The model under review builds one solid part; all positions refer to its coordinate system, in mm. Round coordinates to 2 decimals unless told otherwise and drop trailing zeros. Write each loop counter-clockwise with the first axis right and the second up, starting at its lowest first coordinate (ties: lowest second). Pieces come first, ordered by that corner, then holes. Notation, with made-up numbers: (-26.5, 52) -> (-15.5, 52) arc R11 ccw to (-15.5, 68) -> close; hole circle Ø4 at (-14, 46). An arc over 180 degrees is marked (long way). Return JSON: item names as keys, results as strings. Group by question number.
1. For line 1 along Y through (x, z) = (1, 0); line 2 along Z through (x, y) = (3.55, -1); line 3 along Y through (x, z) = (0.7, 3), list the stretches that pass through material, from the lowest coordinate up. Write a range as from..to.
2. Take a section at D-D, the plane z = -22. Write out the cut boundary in (x, y), then the cut area to 3 significant figures.
3. Take a section at B-B, the plane x = 2.1. Write out the cut boundary in (y, z), then the cut area to 3 significant figures.
4. Take a section at C-C, the plane y = 50. Write out the cut boundary in (x, z), then the cut area to 3 significant figures.
5. Take a section at A-A, the plane z = 0. Write out the cut boundary in (x, y), then the cut area to 3 significant figures.
6. Clearance check with a flat-ended pin moving along its axis: P1, Ø5, axis at y = 14.5, z = 44.5, coming from the -X side. State where the tip first meets the part, or that it passes through.
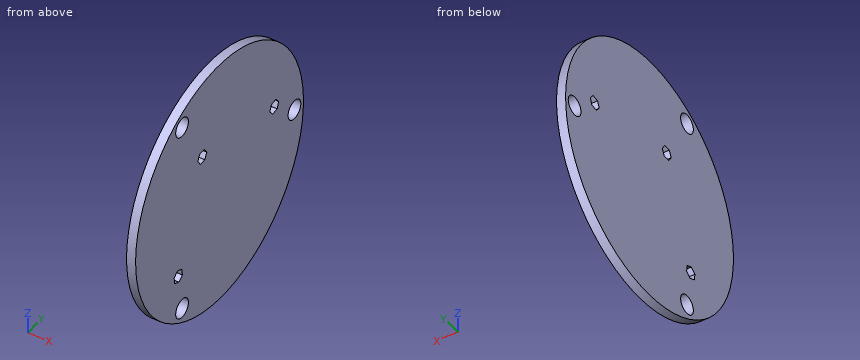
from build123d import *

# Parameters (mm, degrees)
SKETCH1_R           = 56
BOSS_EXTRUDE1_DEPTH = 4
SKETCH2_R           = 4.25
CUT_EXTRUDE1_DEPTH  = 80.296910406
CUT_EXTRUDE3_DEPTH  = 80.296910406


with BuildPart() as part:
    # Sketch1 → Boss-Extrude1 (new body)
    with BuildSketch(Plane(origin=(0, 0, 0), x_dir=(0, 0, -1), z_dir=(1, 0, 0))):
        Circle(SKETCH1_R)
    extrude(amount=BOSS_EXTRUDE1_DEPTH)

    # Sketch2 → Cut-Extrude1 (cut, through all)
    with BuildSketch(Plane.ZY):
        with Locations((0, 50)):
            Circle(SKETCH2_R)
        with Locations((43.301270189, -25)):
            Circle(SKETCH2_R)
        with Locations((-43.301270189, -25)):
            Circle(SKETCH2_R)
    extrude(amount=-CUT_EXTRUDE1_DEPTH, mode=Mode.SUBTRACT)

    # Sketch4 → Cut-Extrude3 (cut, through all)
    with BuildSketch(Plane(origin=(4, 0, 0), x_dir=(0, 0, -1), z_dir=(1, 0, 0))):
        Polygon((27.459399078, -24.776044357), (24.480611991, -25.150424944), (23.315441547, -27.917320527), (25.12905819, -30.309835523), (28.107845277, -29.935454936), (29.273015721, -27.168559353), align=None)
        Polygon((-13.023850584, 34.635102926), (-10.212575655, 33.581505942), (-7.894496437, 35.489342956), (-8.387692148, 38.450776954), (-11.198967077, 39.504373938), (-13.517046295, 37.596536924), align=None)
        Polygon((-17.236572945, -12.849128791), (-17.40919881, -9.85187444), (-20.091210152, -8.502745649), (-22.600595629, -10.150871209), (-22.427969764, -13.14812556), (-19.745958422, -14.497254351), align=None)
    extrude(amount=-CUT_EXTRUDE3_DEPTH, mode=Mode.SUBTRACT)


solid = part.part
Output:
{
 "1": {"line 1": "y = -56..45.75, 54.25..56", "line 2": "z = -55.99..55.99", "line 3": "y = -55.92..46.99, 53.01..55.92"},
 "2": {"outline": "(0, -51.5) -> (4, -51.5) -> (4, 51.5) -> (0, 51.5) -> close", "area": "412 mm^2"},
 "3": {"outline": "circle Ø112 at (0, 0); hole (-30.31, -25.13) -> (-29.94, -28.11) -> (-27.17, -29.27) -> (-24.78, -27.46) -> (-25.15, -24.48) -> (-27.92, -23.32) -> close; hole circle Ø8.5 at (-25, -43.3); hole circle Ø8.5 at (-25, 43.3); hole (-14.5, 19.75) -> (-12.85, 17.24) -> (-9.85, 17.41) -> (-8.5, 20.09) -> (-10.15, 22.6) -> (-13.15, 22.43) -> close; hole (33.58, 10.21) -> (35.49, 7.89) -> (38.45, 8.39) -> (39.5, 11.2) -> (37.6, 13.52) -> (34.64, 13.02) -> close; hole circle Ø8.5 at (50, 0)", "area": "9,610 mm^2"},
 "4": {"outline": "(0, -25.22) -> (4, -25.22) -> (4, -4.25) -> (0, -4.25) -> close; (0, 4.25) -> (4, 4.25) -> (4, 25.22) -> (0, 25.22) -> close", "area": "168 mm^2"},
 "5": {"outline": "(0, -56) -> (4, -56) -> (4, 45.75) -> (0, 45.75) -> close; (0, 54.25) -> (4, 54.25) -> (4, 56) -> (0, 56) -> close", "area": "414 mm^2"},
 "6": {"P1": "stops at x = 0"}
}
